from build123d import *

# Parameters (mm, degrees)
SALIENTE_EXTRUIR1_DEPTH = 10
CROQUIS4_R              = 2
CORTAR_EXTRUIR1_DEPTH   = 23
CROQUIS5_R              = 2
CORTAR_EXTRUIR2_DEPTH   = 23


with BuildPart() as part:
    # Croquis2 → Saliente-Extruir1 (new body)
    with BuildSketch(Plane(origin=(0, 0, 0), x_dir=(0, 0, -1), z_dir=(1, 0, 0))):
        with BuildLine():
            Line((-100, 5), (-100, 0))
            Line((-100, 0), (100, 0))
            Line((100, 0), (100, 5))
            Line((100, 5), (49, 5))
            ThreePointArc((49, 5), (36.752551286, 9.188611699), (29.635083269, 20))
            Line((29.635083269, 20), (39, 20))
            Line((39, 20), (39, 25))
            Line((39, 25), (24.494897428, 25))
            ThreePointArc((24.494897428, 25), (-25, 30), (24.494897428, 35))
            Line((24.494897428, 35), (39, 35))
            Line((39, 35), (39, 40))
            Line((39, 40), (27.221315178, 40))
            ThreePointArc((27.221315178, 40), (-5.078477126, 58.551866315), (-29, 30))
            Line((-29, 30), (-29, 25))
            ThreePointArc((-29, 25), (-34.857864376, 10.857864376), (-49, 5))
            Line((-49, 5), (-100, 5))
        make_face()
    extrude(amount=SALIENTE_EXTRUIR1_DEPTH)

    # Croquis4 → Cortar-Extruir1 (cut)
    with BuildSketch(Plane(origin=(0, 40, 0), x_dir=(1, 0, 0), z_dir=(0, 1, 0))):
        with Locations(Location((5, 33.110657589, 0), (0, 0, 270))):
            Circle(CROQUIS4_R)
    extrude(amount=-CORTAR_EXTRUIR1_DEPTH, mode=Mode.SUBTRACT)

    # Croquis5 → Cortar-Extruir2 (cut)
    with BuildSketch(Plane(origin=(0, 5, 0), x_dir=(1, 0, 0), z_dir=(0, 1, 0))):
        with Locations(Location((5, -92.5, 0), (0, 0, 270))):
            Circle(CROQUIS5_R)
        with Locations(Location((5, 92.5, 0), (0, 0, 270))):
            Circle(CROQUIS5_R)
    extrude(amount=-CORTAR_EXTRUIR2_DEPTH, mode=Mode.SUBTRACT)


solid = part.part
Geometry: final body of the model. Coordinates: model frame, mm. A direction names the side the tool comes from. Coordinates: 2 decimals unless noted, no trailing zeros. Order: outer loops, then holes, each group sorted by start corner. A loop starts at its lowest first (then second) coordinate and runs counter-clockwise, first axis right, second up. Notation, with made-up numbers: (45, 12) - (71, 12) arc R30 ccw to (71, 35) - close; hole circle Ø9 at (61.5, -15). An arc over 180 degrees is marked (long way). Use one line per item in the form item = value.
1) Section C-C (y = 37). Return loops of the section in (x, z), then the cut area to 3 significant figures.
Solutions:
outline = (0, -39) - (10, -39) - (10, -24) - (0, -24) - close; (0, 24) - (10, 24) - (10, 28.14) - (0, 28.14) - close; hole circle Ø4 at (5, -33.11)
area = 179 mm^2
2) Section A-A (x = 5). State how many separate pieces and enclosed holes the cut face has, then the cut area to 3 significant figures.
Solutions:
separate_pieces = 5
enclosed_holes = 0
area = 1,960 mm^2
3) Section D-D (y = 15.5). Return loops of the section in (x, z), then the cut area to 3 significant figures.
Solutions:
outline = (0, -31.4) - (10, -31.4) - (10, -20.37) - (0, -20.37) - close; (0, 20.37) - (10, 20.37) - (10, 31.4) - (0, 31.4) - close
area = 221 mm^2
4) Pin query (flat end, axial travel): pin 1 (5 mm diameter, centred on x = 6, z = 76, fed in from +Y); pin 2 (3 mm diameter, centred on x = 5.5, z = -30.5, fed in from +Y); pin 3 (2.5 mm diameter, centred on x = 5, z = -33.11, fed in from +Y); pin 4 (4.5 mm diameter, centred on x = 5, z = -33.11, fed in from -Y). Return the tip coordinate at first contact, or that it passes through.
Solutions:
pin_1 = 5
pin_2 = 40
pin_3 = 14.69
pin_4 = 0
5) Set-up query: faces 1 (the face through (2.7, 40, -33.2)), 2 (the face through (5, 25, -30)), 3 (the face through (5, 28, 29)). Return all of +Z, -Z, +X, -X, +Y, -Y with unobstructed straight access to the full face (end or side cutting, diameter ignored); none if empty.
Solutions:
face_1 = -Z, +X, -X, +Y
face_2 = -Z, +X, -X
face_3 = +Z, +X, -X, +Y
6) Ray query, L1, parallel to Z at x = 5.25, y = 22; L2, parallel to Y at x = 7, z = 0; L3, parallel to Y at x = 7, z = 85.5. Return the intervals inside material, ascending.
Solutions:
L1 = -39 to -35.09, -31.13 to -23.69, 23.69 to 29.23
L2 = 0 to 5, 55 to 59
L3 = 0 to 5
7) Section B-B (z = 92.5). Return loops of the section in (x, y).
Solutions:
outline = (0, 0) - (3, 0) - (3, 5) - (0, 5) - close; (7, 0) - (10, 0) - (10, 5) - (7, 5) - close
8) Mould query, pull axis X, two halves, no side actions, for faces 4 (the face through (10, 5.6, -6.9)), 5 (the face through (5, 5, -75)), 6 (the face through (5.09, 37.53, -35.11)). Classes: +X half, -X half, draft (parallel to the pull), parting line (faces both ways), or undercut.
Solutions:
face_4 = +X half
face_5 = draft
face_6 = undercut
